Geometry: final body of the model. Coordinates: model frame, mm. A direction names the side the tool comes from. Give positions to 0.01 mm unless a question says otherwise; leave off trailing zeros. Write each loop counter-clockwise with the first axis right and the second up, starting at its lowest first coordinate (ties: lowest second). Pieces come first, ordered by that corner, then holes. Notation, with made-up numbers: M 3,70 L 22,70 A31 cw 22,98 Z; hole C 8.5,0.5 d7. An arc over 180 degrees is marked long. Answer as a JSON object with one key per item and string values.
from build123d import *

# Parameters (mm, degrees)
SKETCH_1_W          = 42
SKETCH_1_H          = 42
SKETCH_1_R          = 1.5
EXTRUDE_1_DEPTH     = 5
SKETCH_2_W          = 42
SKETCH_2_H          = 6
EXTRUDE_2_DEPTH     = 65
CUT_EXTRUDE_2_DEPTH = 65
SKETCH_4_R          = 11.5
CUT_EXTRUDE_3_DEPTH = 10


with BuildPart() as part:
    # 草图1 → 凸台-拉伸1 (new body)
    with BuildSketch(Plane(origin=(0, 0, 0), x_dir=(0, 0, -1), z_dir=(1, 0, 0))):
        with Locations((-27.709265176, 0)):
            Rectangle(SKETCH_1_W, SKETCH_1_H)
        with Locations((-12.209265176, 15.5)):
            Circle(SKETCH_1_R, mode=Mode.SUBTRACT)
        with Locations((-43.209265176, 15.5)):
            Circle(SKETCH_1_R, mode=Mode.SUBTRACT)
        with Locations((-12.209265176, -15.5)):
            Circle(SKETCH_1_R, mode=Mode.SUBTRACT)
        with Locations((-43.209265176, -15.5)):
            Circle(SKETCH_1_R, mode=Mode.SUBTRACT)
    extrude(amount=EXTRUDE_1_DEPTH)

    # 草图2 → 凸台-拉伸2 (add)
    with BuildSketch(Plane.ZY):
        with Locations((27.709265176, -24)):
            Rectangle(SKETCH_2_W, SKETCH_2_H)
    extrude(amount=-EXTRUDE_2_DEPTH)

    # 草图3 → 切除-拉伸2 (cut)
    with BuildSketch(Plane(origin=(0, -27, 0), x_dir=(-1, 0, 0), z_dir=(0, -1, 0))):
        with BuildLine():
            ThreePointArc((-55, -35.722195546), (-57.48706963, -38.209265176), (-55, -40.696334806))
            Line((-55, -40.696334806), (-55, -35.722195546))
        make_face()
        with BuildLine():
            Line((-55, -35.722195546), (-55, -40.696334806))
            ThreePointArc((-55, -40.696334806), (-53.241376199, -39.967888976), (-52.51293037, -38.209265176))
            ThreePointArc((-52.51293037, -38.209265176), (-53.241376199, -36.450641375), (-55, -35.722195546))
        make_face()
        with BuildLine():
            Line((-55, -40.709265176), (-10, -40.709265176))
            ThreePointArc((-10, -40.709265176), (-12.5, -38.209265176), (-10, -35.709265176))
            Line((-10, -35.709265176), (-55, -35.709265176))
            Line((-55, -35.709265176), (-55, -35.722195546))
            ThreePointArc((-55, -35.722195546), (-53.241376199, -36.450641375), (-52.51293037, -38.209265176))
            ThreePointArc((-52.51293037, -38.209265176), (-53.241376199, -39.967888976), (-55, -40.696334806))
            Line((-55, -40.696334806), (-55, -40.709265176))
        make_face()
        with BuildLine():
            ThreePointArc((-10, -35.709265176), (-12.5, -38.209265176), (-10, -40.709265176))
            Line((-10, -40.709265176), (-10, -35.709265176))
        make_face()
        with BuildLine():
            Line((-10, -35.709265176), (-10, -40.709265176))
            ThreePointArc((-10, -40.709265176), (-8.232233047, -39.977032129), (-7.5, -38.209265176))
            ThreePointArc((-7.5, -38.209265176), (-8.232233047, -36.441498223), (-10, -35.709265176))
        make_face()
        with BuildLine():
            ThreePointArc((-10, -14.709265176), (-12.5, -17.209265176), (-10, -19.709265176))
            Line((-10, -19.709265176), (-10, -14.709265176))
        make_face()
        with BuildLine():
            Line((-10, -14.709265176), (-10, -19.709265176))
            ThreePointArc((-10, -19.709265176), (-8.232233047, -18.977032129), (-7.5, -17.209265176))
            ThreePointArc((-7.5, -17.209265176), (-8.232233047, -15.441498223), (-10, -14.709265176))
        make_face()
        with BuildLine():
            Line((-55, -19.709265176), (-10, -19.709265176))
            ThreePointArc((-10, -19.709265176), (-12.5, -17.209265176), (-10, -14.709265176))
            Line((-10, -14.709265176), (-55, -14.709265176))
            Line((-55, -14.709265176), (-55, -14.722195546))
            ThreePointArc((-55, -14.722195546), (-53.241376199, -15.450641375), (-52.51293037, -17.209265176))
            ThreePointArc((-52.51293037, -17.209265176), (-53.241376199, -18.967888976), (-55, -19.696334806))
            Line((-55, -19.696334806), (-55, -19.709265176))
        make_face()
        with BuildLine():
            ThreePointArc((-55, -14.722195546), (-57.48706963, -17.209265176), (-55, -19.696334806))
            Line((-55, -19.696334806), (-55, -14.722195546))
        make_face()
        with BuildLine():
            Line((-55, -14.722195546), (-55, -19.696334806))
            ThreePointArc((-55, -19.696334806), (-53.241376199, -18.967888976), (-52.51293037, -17.209265176))
            ThreePointArc((-52.51293037, -17.209265176), (-53.241376199, -15.450641375), (-55, -14.722195546))
        make_face()
    extrude(amount=-CUT_EXTRUDE_2_DEPTH, mode=Mode.SUBTRACT)

    # 草图4 → 切除-拉伸3 (cut)
    with BuildSketch(Plane(origin=(5, 0, 0), x_dir=(0, 0, -1), z_dir=(1, 0, 0))):
        with Locations((-27.709265176, 0)):
            Circle(SKETCH_4_R)
    extrude(amount=-CUT_EXTRUDE_3_DEPTH, mode=Mode.SUBTRACT)


solid = part.part
1) Line query: line 1 (Z direction, x = 55.5, y = -21.5); line 2 (Z direction, x = 3, y = -15); line 3 (Y direction, x = 47, z = 14). Output: solid intervals per line, ascending. Write a range as from..to.
Geometry check:
{"line 1": "z = 6.71..14.77, 19.65..35.77, 40.65..48.71", "line 2": "z = 6.71..10.8, 13.62..41.8, 44.62..48.71", "line 3": "y = -27..-21"}
2) Cut plane D-D on z = 22. Return loops of the section in (x, y).
Geometry check:
{"outline": "M 0,-27 L 65,-27 L 65,-21 L 5,-21 L 5,-9.98 L 0,-9.98 Z; M 0,9.98 L 5,9.98 L 5,21 L 0,21 Z"}
3) Pull-direction query (Z, two-part tool) for faces 4 (the flat face through (23, -23, 6.709)), 5 (the flat face through (65, -24, 27)), 6 (the cylindrical face through (57.486, -24.042, 38.155)); classes: pulls with the +Z half, pulls with the -Z half, needs draft (parallel to the pull), parting line crosses it, or undercut.
Geometry check:
{"face 4": "pulls with the -Z half", "face 5": "needs draft", "face 6": "undercut"}
4) Set-up query: faces 1 (the flat face through (35, -21, 27)), 2 (the cylindrical face through (2.465, 15.566, 13.708)), 3 (the flat face through (33, -24, 19.709)). Return all of +Z, -Z, +X, -X, +Y, -Y with unobstructed straight access to the full face (end or side cutting, diameter ignored); none if empty.
Geometry check:
{"face 1": "+Z, -Z, +X, +Y", "face 2": "+X, -X", "face 3": "+Y, -Y"}
5) Cut plane B-B on x = 54. Return loops of the section in (y, z), and give its area (3 significant figures).
Geometry check:
{"outline": "M -27,6.71 L -21,6.71 L -21,14.71 L -27,14.71 Z; M -27,19.71 L -21,19.71 L -21,35.71 L -27,35.71 Z; M -27,40.71 L -21,40.71 L -21,48.71 L -27,48.71 Z", "area": "192 mm2"}
6) Cut plane C-C on y = 0. Return loops of the section in (x, z), and give its area (3 significant figures).
Geometry check:
{"outline": "M 0,6.71 L 5,6.71 L 5,16.21 L 0,16.21 Z; M 0,39.21 L 5,39.21 L 5,48.71 L 0,48.71 Z", "area": "95.0 mm2"}
7) Contact query for flat-ended pins moving along their axis: P1, Ø6, axis at x = 21.5, z = 22.5, coming from the +Y side; P2, Ø21, axis at y = -0.5, z = 23, coming from the +X side. Output: stop coordinate, or through.
Geometry check:
{"P1": "stops at y = -21", "P2": "stops at x = 5"}
8) Cut plane A-A on y = -15.5. Return loops of the section in (x, z), and give its area (3 significant figures).
Geometry check:
{"outline": "M 0,6.71 L 5,6.71 L 5,10.71 L 0,10.71 Z; M 0,13.71 L 5,13.71 L 5,41.71 L 0,41.71 Z; M 0,44.71 L 5,44.71 L 5,48.71 L 0,48.71 Z", "area": "180 mm2"}
